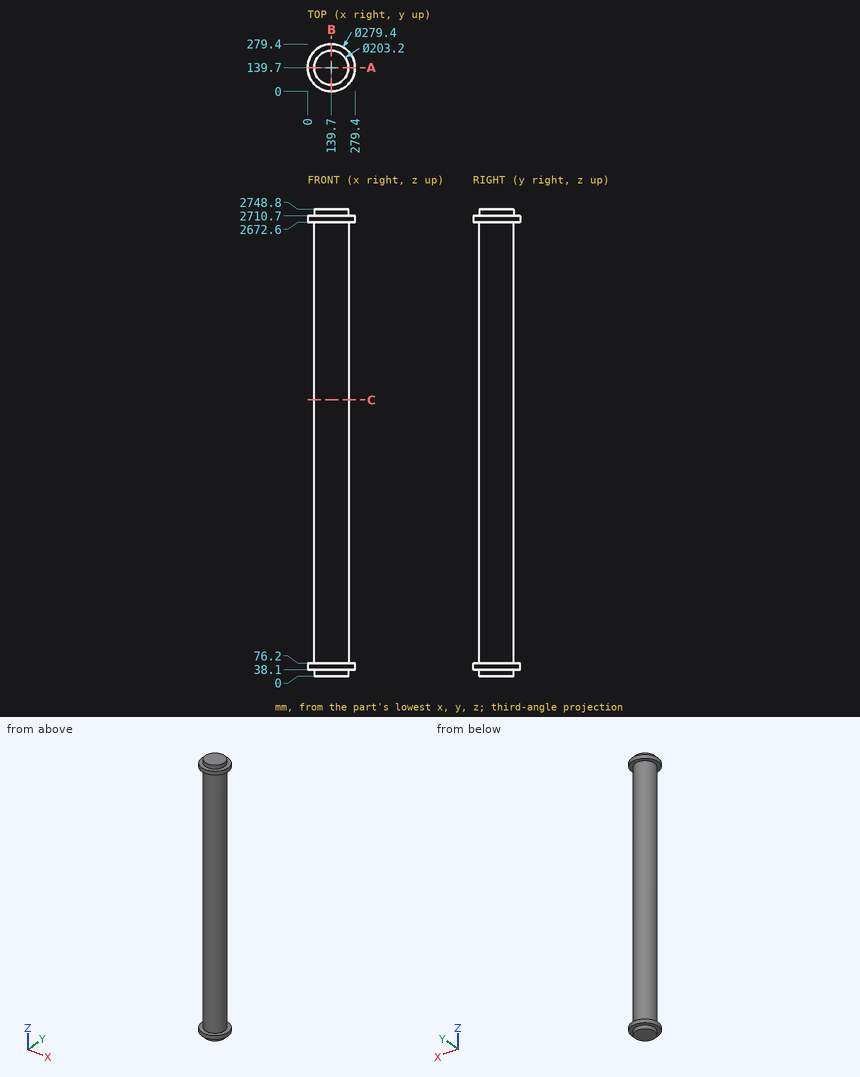
Check sheet for the drawn part. Datum: minimum x, y, z corner. Units: mm. Round coordinates to 2 decimals unless told otherwise and drop trailing zeros. Loops run counter-clockwise (first coordinate to the right, second up) from the corner with the lowest first, then second, coordinate; pieces in that order, holes last. Notation, with made-up numbers: (74, 81.5) - (95, 81.5) arc R27 ccw to (95, 105.5) - close; hole circle Ø6 at (5, 3). An arc over 180 degrees is marked (long way). Answer as a JSON object with one key per item and string values. Group by question number.
Q1. Sectioned sample at C-C, the plane z = 1627. Enter the section's corners in (x, y), plus the area to 3 significant figures.
Q2. Sectioned sample at A-A, the plane y = 139.7. Enter the section's corners in (x, z), plus the area to 3 significant figures.
Q3. Scan lines: line 1 along Z through (x, y) = (54, 219); line 2 along Y through (x, z) = (135, 1942); line 3 along X through (y, z) = (142, 1104). Record each from-to range of solid material in increasing order. Write a range as [from, to].
Q4. Gauge pin test, flat ends, axial feed: P1, Ø6, axis at y = 166, z = 995.5, coming from the -X side; P2, Ø6, axis at y = 58, z = 2452.5, coming from the +X side; P3, Ø4, axis at x = 158, z = 445, coming from the -Y side. Record the tip position at first contact, or that the pin passes through.
Solution:
{
 "1": {"outline": "circle Ø203.2 at (139.7, 139.7)", "area": "32,400 mm²"},
 "2": {"outline": "(0, 38.1) - (38.1, 38.1) - (38.1, 0) - (241.3, 0) - (241.3, 38.1) - (279.4, 38.1) - (279.4, 76.2) - (241.3, 76.2) - (241.3, 2672.6) - (279.4, 2672.6) - (279.4, 2710.7) - (241.3, 2710.7) - (241.3, 2748.8) - (38.1, 2748.8) - (38.1, 2710.7) - (0, 2710.7) - (0, 2672.6) - (38.1, 2672.6) - (38.1, 76.2) - (0, 76.2) - close", "area": "564,000 mm²"},
 "3": {"line 1": "z = [38.1, 76.2], [2672.6, 2710.7]", "line 2": "y = [38.21, 241.19]", "line 3": "x = [38.13, 241.27]"},
 "4": {"P1": "stops at x = 40.81", "P2": "stops at x = 203.96", "P3": "stops at y = 39.42"}
}
